Input: part model. Units: mm. Frame: model coordinates. A direction names the side the tool comes from. Round coordinates to 2 decimals unless told otherwise and drop trailing zeros. Order: outer loops, then holes, each group sorted by start corner. A loop starts at its lowest first (then second) coordinate and runs counter-clockwise, first axis right, second up. Notation, with made-up numbers: M 71,5.25 L 81,5.25 A8 cw 81,10.25 Z; hole C 55.5,85.25 d8. An arc over 180 degrees is marked long. One line per question, with ' | ' between items.
Autodesk Inventor part; units mm, degrees
ref_plane "Work Plane1" through (0, 0, 603.25) normal (0, 0, -1) x (-1, 0, 0)
ref_plane "YZ Plane" through (0, 0, 0) normal (1, 0, 0) x (0, 1, 0)
ref_plane "XZ Plane" through (0, 0, 0) normal (0, 1, 0) x (-1, 0, 0)
sketch "Sketch1" plane through (0, 0, 0) normal (0, 0, 1) x (1, 0, 0)
  line L0 (0, 6.2128) -> (0, 95.3872)
  line L1 (6.2128, 101.6) -> (146.1872, 101.6)
  line L2 (152.4, 95.3872) -> (152.4, 6.2128)
  line L3 (149.3622, 6.2128) -> (149.3622, 95.3872)
  line L4 (146.1872, 98.5622) -> (6.2128, 98.5622)
  line L5 (3.0378, 95.3872) -> (3.0378, 6.2128)
  arc A0 (6.2128, 98.5622) -> (3.0378, 95.3872) centre (6.2128, 95.3872) ccw
  arc A1 (149.3622, 95.3872) -> (146.1872, 98.5622) centre (146.1872, 95.3872) ccw
  arc A2 (6.2128, 101.6) -> (0, 95.3872) centre (6.2128, 95.3872) ccw
  arc A3 (152.4, 95.3872) -> (146.1872, 101.6) centre (146.1872, 95.3872) ccw
  line L6 (-101.6, 0) -> (-3.175, 0)
  line L7 (-3.175, 3.0378) -> (-101.6, 3.0378)
  line L8 (-101.6, 3.0378) -> (-101.6, 0)
  line L9 (254, 0) -> (155.575, 0)
  line L10 (155.575, 3.0378) -> (254, 3.0378)
  line L11 (254, 3.0378) -> (254, 0)
  arc A4 (-3.175, 3.0378) -> (0, 6.2128) centre (-3.175, 6.2128) ccw
  arc A5 (152.4, 6.2128) -> (155.575, 3.0378) centre (155.575, 6.2128) ccw
  arc A6 (-3.175, 0) -> (3.0378, 6.2128) centre (-3.175, 6.2128) ccw
  arc A7 (149.3622, 6.2128) -> (155.575, 0) centre (155.575, 6.2128) ccw
  point P0 (0, 0)
  point P1 (0, 101.6)
  point P2 (152.4, 101.6)
  point P3 (152.4, 3.0378)
  point P4 (149.3622, 0)
  dimension "d0" = 101.6
  dimension "d1" = 3.0378
  dimension "d2" = 3.0378
  dimension "d3" = 152.4
  dimension "d4" = 3.175
  dimension "d5" = 6.2128
  dimension "d31" = 3.0378
  dimension "d32" = 3.0378
  dimension "d33" = 3.175
  dimension "d34" = 6.2128
  dimension "d35" = 101.6
extrude "Extrusion1" add sketch "Sketch1" along normal blind 1206.5
hole "Hole1" at (25.4, 101.6, 1130.3) direction (0, -1, 0) diameter 9.906 end through all
pattern_linear "Rectangular Pattern1" count 2 spacing 31.75 along (1, 0, 0) of "Hole1"
pattern_linear "Rectangular Pattern2" count 2 spacing 1054.1 along (0, 0, -1) of "Hole1", "Rectangular Pattern1"
sketch "Sketch3" plane through (6.2128, 101.6, 0) normal (0, 1, 0) x (1, 0, 0)
  line L0 (0, -1206.5) -> (139.9743, -1206.5)
  line L1 (19.1872, -698.5) -> (120.7872, -698.5)
  line L2 (127.1372, -692.15) -> (127.1372, -501.65)
  line L3 (120.7872, -495.3) -> (19.1872, -495.3)
  line L4 (12.8372, -501.65) -> (12.8372, -692.15)
  arc A0 (12.8372, -692.15) -> (19.1872, -698.5) centre (19.1872, -692.15) ccw
  arc A1 (19.1872, -495.3) -> (12.8372, -501.65) centre (19.1872, -501.65) ccw
  arc A2 (127.1372, -501.65) -> (120.7872, -495.3) centre (120.7872, -501.65) ccw
  arc A3 (120.7872, -698.5) -> (127.1372, -692.15) centre (120.7872, -692.15) ccw
  line L5 (146.1872, 0) -> (146.1872, -1206.5)
  point P0 (-6.2128, 0)
  dimension "d36" = 6.35
  dimension "d37" = 203.2
  dimension "d38" = 114.3
  dimension "d39" = 19.05
  dimension "d40" = 508
extrude "Extrusion2" cut sketch "Sketch3" against normal blind 25.4
sketch "Sketch4" plane through (6.2128, 101.6, 0) normal (0, 1, 0) x (1, 0, 0)
  line L0 (0, -1206.5) -> (139.9743, -1206.5)
  line L1 (139.9743, 0) -> (139.9743, -1206.5)
  line L2 (0, 0) -> (0, -1206.5)
  line L3 (63.6372, -1092.2) -> (76.3372, -1092.2)
  line L4 (82.6872, -1085.85) -> (82.6872, -1063.625)
  line L5 (76.3372, -1057.275) -> (63.6372, -1057.275)
  line L6 (57.2872, -1063.625) -> (57.2872, -1085.85)
  arc A0 (57.2872, -1085.85) -> (63.6372, -1092.2) centre (63.6372, -1085.85) ccw
  arc A1 (76.3372, -1092.2) -> (82.6872, -1085.85) centre (76.3372, -1085.85) ccw
  arc A2 (82.6872, -1063.625) -> (76.3372, -1057.275) centre (76.3372, -1063.625) ccw
  arc A3 (63.6372, -1057.275) -> (57.2872, -1063.625) centre (63.6372, -1063.625) ccw
  point P0 (-6.2128, 0)
  point P1 (57.2872, -1092.2)
  point P2 (82.6872, -1057.275)
  point P3 (57.2872, -1057.275)
  dimension "d43" = 114.3
  dimension "d44" = 57.2872
  dimension "d45" = 25.4
  dimension "d46" = 139.9743
  dimension "d47" = 34.925
  dimension "d48" = 6.35
extrude "Extrusion3" cut sketch "Sketch4" against normal blind 25.4
hole "Hole2" at (88.9, 101.6, 1041.4) direction (0, -1, 0) diameter 4.826 depth 25.4 tip angle 118
pattern_linear "Rectangular Pattern3" count 2 spacing 25.4 along (-1, 0, 0) of "Hole2"
ref_plane "Work Plane1" through (0, 0, 603.25) normal (0, 0, -1) x (-1, 0, 0)
mirror "Mirror1" about plane through (0, 0, 603.25) normal (0, 0, -1) of "Extrusion3", "Hole2", "Rectangular Pattern3"
equation "\"d2\" = d1"
equation "\"d5\" = d4 + d1"
equation "\"d31\" = d1"
equation "\"d32\" = d1"
equation "\"d33\" = d4"
equation "\"d34\" = d5"
equation "\"d44\" = -0.5 * d45 + 0.5 * d46"
properties part number "GE-12021" material "Steel"
Item 1: Line query: line 1 along Z through (x, y) = (57, 100); line 2 along X through (y, z) = (73.5, 336); line 3 along X through (y, z) = (100, 1041). Output: solid intervals per line, ascending. Write a range as from..to.
Report:
line 1: 0..71.25, 81.15..495.3, 698.5..1125.35, 1135.25..1206.5 | line 2: 0..3.04, 149.36..152.4 | line 3: 2.05..61.12, 65.88..86.52, 91.28..150.35
Item 2: Section query A-A, the plane y = 74. Return loops of the section in (x, z).
Report:
outline: M 0,0 L 3.04,0 L 3.04,1206.5 L 0,1206.5 Z; M 149.36,0 L 152.4,0 L 152.4,1206.5 L 149.36,1206.5 Z
Item 3: Section query B-B, the plane z = 796.5. Return loops of the section in (x, y) (3 decimals).
Report:
outline: M -101.6,0 L -3.175,0 A6.213 ccw 3.038,6.213 L 3.038,95.387 A3.175 cw 6.213,98.562 L 146.187,98.562 A3.175 cw 149.362,95.387 L 149.362,6.213 A6.213 ccw 155.575,0 L 254,0 L 254,3.038 L 155.575,3.038 A3.175 cw 152.4,6.213 L 152.4,95.387 A6.213 ccw 146.187,101.6 L 6.213,101.6 A6.213 ccw 0,95.387 L 0,6.213 A3.175 cw -3.175,3.038 L -101.6,3.038 Z
Item 4: Section query C-C, the plane x = 209.5. Return loops of the section in (y, z), plus the area to 3 significant figures.
Report:
outline: M 0,0 L 3.04,0 L 3.04,1206.5 L 0,1206.5 Z | area: 3,670 mm²
Item 5: Mould query, pull axis X, two halves, no side actions, for faces 6 (the flat face through (-53, 0, 595)), 7 (the flat face through (152.4, 51, 595)), 8 (the flat face through (3.038, 51, 595)). Classes: +X half, -X half, draft (parallel to the pull), parting line (faces both ways), or undercut.
Report:
face 6: draft | face 7: +X half | face 8: undercut
Item 6: First-contact query: pin 1 (5 mm diameter, centred on y = 13, z = 933, fed in from -X); pin 2 (3 mm diameter, centred on x = 88.9, z = 165.1, fed in from +Y); pin 3 (1.5 mm diameter, centred on y = 99.5, z = 127, fed in from +X); pin 4 (1.5 mm diameter, centred on y = 100.5, z = 629.5, fed in from +X). Flat tips, straight axial feed; report the tip coordinate or a pass-through.
Report:
pin 1: x = 0 | pin 2: through | pin 3: x = 151.41 | pin 4: x = 150.61
Item 7: Access query for faces 1 (the flat face through (204, 3.038, 595)), 2 (the flat face through (0, 50, 595)), 3 (the flat face through (205, 0, 595)), 4 (the flat face through (139, 98.562, 595)), 5 (the flat face through (137, 101.6, 595)). Directions: +Z, -Z, +X, -X, +Y, -Y. A direction counts if a zero-diameter tool reaches every point of the face in a straight line with its end or side. Return the directions, or none.
Report:
face 1: +Z, -Z, +X, +Y | face 2: +Z, -Z, -X, +Y | face 3: +Z, -Z, +X, -X, -Y | face 4: +Z, -Z, -Y | face 5: +Z, -Z, +X, -X, +Y
